For this review, take the finished solid that the model builds, in its own axes (mm). A direction names the side the tool comes from. Round coordinates to 2 decimals unless told otherwise and drop trailing zeros. Order: outer loops, then holes, each group sorted by start corner. A loop starts at its lowest first (then second) coordinate and runs counter-clockwise, first axis right, second up. Notation, with made-up numbers: (68, 48) -> (82, 48) arc R13 ccw to (82, 60) -> close; hole circle Ø11 at (19, 70). An arc over 180 degrees is marked (long way). Use a Markdown table: item, result. Add a question column.
1) Draft analysis for pull direction Y (two halves, no side actions). For faces 5 (the face through (42, -35.5, 10)), 6 (the face through (15.145, -33.007, 13.498)), 7 (the face through (43, 30.8, 12)), state which applies: pulls with the +Y half, pulls with the -Y half, needs draft (parallel to the pull), parting line crosses it, or undercut.
2) Machinability: for faces 1 (the face through (41, -22.3, 5)), 2 (the face through (13.81, 0.25, 3.97)), 3 (the face through (62, -29, 15)), 4 (the face through (62.3, -19, 2)), which of the approach directions +Z, -Z, +X, -X, +Y, -Y give a long, thin tool a straight path to every point of the face, cutting with its end or side? Answer none if there is none.
3) Wall thickness on line 1 along Y through (x, z) = (17, 1.7); line 2 along Y through (x, z) = (31.5, 14.5); line 3 along Y through (x, z) = (33.5, 2): over which ranges is each line inside the solid? List them lowest first. Write a range as [from, to].
4) Consider section A-A (x = 46). State the section outline as (y, z) points.
5) Consider section B-B (y = 8.5). Give the number of separate pieces and of enclosed holes in the cut face, plus the area to 3 significant figures.
6) Clearance check with flat-ended pins moving along their axes: P1, Ø6.5, axis at y = -12, z = 3, coming from the +X side; P2, Ø12, axis at y = 15.5, z = 4.5, coming from the +X side; P3, Ø6.5, axis at x = 18.5, y = -24, coming from the +Z side; P4, Ø8, axis at x = 66.5, y = -1.5, coming from the +Z side. State where each tip first meets the part, or that it passes through.
```python
from build123d import *

# Parameters (mm, degrees)
SKETCH009_R     = 1.75
PAD001_DEPTH    = 21
POCKET008_DEPTH = 35.5010001
POCKET009_DEPTH = 15
POCKET010_DEPTH = 18
SKETCH013_W     = 2
SKETCH013_H     = 12.5
POCKET011_DEPTH = 4
POCKET012_DEPTH = 3
POCKET013_DEPTH = 3.05
POCKET017_DEPTH = 3
SKETCH021_R     = 3
POCKET018_DEPTH = 3


with BuildPart() as part:
    # Sketch009 → Pad001 (new body)
    with BuildSketch(Plane.XY):
        with BuildLine():
            Line((11, 0), (23.3, 0))
            Line((23.3, 0), (23.3, 22.3))
            Line((23.3, 22.3), (59.9, 22.3))
            Line((59.9, 22.3), (59.9, 10.55))
            Line((59.9, 10.55), (72.15, 10.55))
            Line((72.15, 10.55), (72.15, 0))
            Line((72.15, 0), (80.25, 0))
            ThreePointArc((80.25, 0), (82, 1.75), (83.75, 0))
            Line((83.75, 0), (92, 0))
            add(Edge.make_bspline(
                [(92, 0), (92.391037, 11.810127), (88.126587, 35.076866), (64.2, 35.5)],
                knots=[0, 0, 0, 0, 1, 1, 1, 1], degree=3))
            Line((64.2, 35.5), (20.1, 35.5))
            add(Edge.make_bspline(
                [(0.75, 22.55), (0.790433, 24.50555), (2.8995135699, 28.3383927733), (10.6468681476, 35.231617337), (14.5053016695, 34.8194742751), (20.1, 35.5)],
                knots=[0, 0, 0, 0, 0.3333333333, 0.6666666667, 1, 1, 1, 1], degree=3))
            Line((0.75, 22.55), (0.05, 7.2))
            ThreePointArc((0.05, 7.2), (0.0125001507, 3.6000868045), (0, 0))
            Line((0, 0), (5.5, 0))
            Line((5.5, 0), (5.5, 18))
            Line((5.5, 18), (11, 18))
            Line((11, 18), (11, 0))
        make_face()
        with Locations((17, 25)):
            Circle(SKETCH009_R, mode=Mode.SUBTRACT)
    extrude(amount=PAD001_DEPTH)

    # Sketch010 (on Face1 of Pad001) → Pocket008 (cut, through all)
    with BuildSketch(Plane.XZ):
        with BuildLine():
            Line((7.9, 5), (0, 5))
            Line((0, 5), (0, 21))
            Line((0, 21), (20.05, 21))
            ThreePointArc((20.05, 21), (18.8992105015, 20.6660901767), (18.1058720895, 19.7680777024))
            Line((18.1058720895, 19.7680777024), (12.1, 7.05))
            add(Edge.make_bspline(
                [(12.1, 7.05), (11.7904723155, 6.5431449633), (11.5915441331, 5.8310211118), (9.732416, 5.34755), (7.9, 5)],
                knots=[0, 0, 0, 0, 0.5, 1, 1, 1, 1], degree=3))
        make_face()
    extrude(amount=-POCKET008_DEPTH, mode=Mode.SUBTRACT)

    # Sketch011 (on Face4 of Pocket008) → Pocket009 (cut)
    with BuildSketch(Plane.XY.offset(21)):
        with BuildLine():
            Line((11, 30.8), (11, 0))
            Line((11, 0), (23.3, 0))
            Line((23.3, 0), (23.3, 22.3))
            Line((23.3, 22.3), (59.9, 22.3))
            Line((59.9, 22.3), (59.9, 10.55))
            Line((59.9, 10.55), (72.15, 10.55))
            Line((72.15, 10.55), (72.15, 0))
            Line((72.15, 0), (73.35, 0))
            Line((73.35, 27.75), (73.35, 0))
            Line((73.35, 27.75), (25.4, 27.75))
            ThreePointArc((24.2, 28.95), (24.5514718626, 28.1014718626), (25.4, 27.75))
            Line((24.2, 28.95), (24.2, 30.8))
            Line((24.2, 30.8), (11, 30.8))
        make_face()
    extrude(amount=-POCKET009_DEPTH, mode=Mode.SUBTRACT)

    # Sketch012 (on Face1 of Pocket009) → Pocket010 (cut)
    with BuildSketch(Plane.XZ):
        Polygon((16.7, 6), (11, 6), (11, 2), align=None)
    extrude(amount=-POCKET010_DEPTH, mode=Mode.SUBTRACT)

    # Sketch013 (on Face2 of Pocket010) → Pocket011 (cut)
    with BuildSketch(Plane(origin=(0, 0, 0), x_dir=(1, 0, 0), z_dir=(0, 0, -1))):
        Polygon((72.15, -10.55), (59.9, -10.55), (59.9, -22.3), (23.3, -22.3), (23.3, -24.5), (62.3, -24.5), (62.3, -12.55), (75.35, -12.55), (75.35, 0), (72.15, 0), align=None)
        with Locations((22.3, -6.25)):
            Rectangle(SKETCH013_W, SKETCH013_H)
    extrude(amount=-POCKET011_DEPTH, mode=Mode.SUBTRACT)

    # Sketch014 (on Face36 of Pocket011) → Pocket012 (cut)
    with BuildSketch(Plane.XY.offset(21)):
        with BuildLine():
            Line((73.35, 27.75), (73.35, 0))
            Line((73.35, 0), (89.95, 0))
            add(Edge.make_bspline(
                [(89.95, 0), (89.796112, 11.583797), (90.425743, 22.81332), (73.35, 27.75)],
                knots=[0, 0, 0, 0, 1, 1, 1, 1], degree=3))
        make_face()
    extrude(amount=-POCKET012_DEPTH, mode=Mode.SUBTRACT)

    # Sketch015 (on Face29 of Pocket012) → Pocket013 (cut)
    with BuildSketch(Plane.XZ.offset(-27.75)):
        Polygon((24.2, 6), (73.35, 6), (73.35, 15), (51, 15), (48.45, 16), (25, 16), (24.2, 16.4), align=None)
    extrude(amount=-POCKET013_DEPTH, mode=Mode.SUBTRACT)

    # Sketch020 (on Face36 of Pocket013) → Pocket017 (cut)
    with BuildSketch(Plane.XY.offset(18)):
        with BuildLine():
            ThreePointArc((85, 0), (82, 3), (79, 0))
            Line((79, 0), (85, 0))
        make_face()
    extrude(amount=-POCKET017_DEPTH, mode=Mode.SUBTRACT)

    # Sketch021 (on Face6 of Pocket017) → Pocket018 (cut)
    with BuildSketch(Plane.XY.offset(6)):
        with Locations((17, 25)):
            Circle(SKETCH021_R)
    extrude(amount=-POCKET018_DEPTH, mode=Mode.SUBTRACT)

    # Mirrored: part across XZ


with BuildPart() as part_1:
    add(part.part)
    add(part.part.mirror(Plane.XZ))


solid = part_1.part
```
Results list:
| question | item | result |
|---|---|---|
| 1 | face 5 | pulls with the -Y half |
| 1 | face 6 | needs draft |
| 1 | face 7 | undercut |
| 2 | face 1 | +Z, -Z |
| 2 | face 2 | +Z |
| 2 | face 3 | -X |
| 2 | face 4 | -Z |
| 3 | line 1 | [-35.17, -26.75], [-23.25, 23.25], [26.75, 35.17] |
| 3 | line 2 | [-35.5, -30.8], [30.8, 35.5] |
| 3 | line 3 | [-35.5, -24.5], [24.5, 35.5] |
| 4 | outline | (-35.5, 0) -> (-24.5, 0) -> (-24.5, 4) -> (-22.3, 4) -> (-22.3, 6) -> (-30.8, 6) -> (-30.8, 16) -> (-27.75, 16) -> (-27.75, 21) -> (-35.5, 21) -> close; (22.3, 4) -> (24.5, 4) -> (24.5, 0) -> (35.5, 0) -> (35.5, 21) -> (27.75, 21) -> (27.75, 16) -> (30.8, 16) -> (30.8, 6) -> (22.3, 6) -> close |
| 5 | separate pieces | 3 |
| 5 | enclosed holes | 0 |
| 5 | area | 408 mm2 |
| 6 | P1 | x = 91.47 |
| 6 | P2 | x = 91.36 |
| 6 | P3 | z = 6 |
| 6 | P4 | through |
